Part model, mm, in its own coordinate system. A direction names the side the tool comes from. Round coordinates to 2 decimals unless told otherwise and drop trailing zeros. Write each loop counter-clockwise with the first axis right and the second up, starting at its lowest first coordinate (ties: lowest second). Pieces come first, ordered by that corner, then holes.
1) Saw through at D-D on y = -181. Write the cut outline in (x, z), and give its area (3 significant figures).
2) Which spindle directions (+Z, -Z, +X, -X, +Y, -Y) get a long thin tool onto all of the face, cutting with end or side? Do faces 4 (the flat face through (-100, -8.457, 10)), 5 (the flat face through (-102.851, 20.437, 9.86)), 6 (the flat face through (-12, -99, 20)). Say none if no direction does.
3) Drill centre lines: L1, parallel to Y at x = -142.5, z = 9; L2, parallel to X at y = -266, z = 16.5; L3, parallel to X at y = -232, z = 15.75. Where is each one in solid material? Low to high.
4) Saw through at C-C on x = -182.5. Write the cut outline in (y, z).
5) Saw through at B-B on y = -259. Write the cut outline in (x, z).
6) Flat gauge pins, fed straight in: pin 1 (1 mm diameter, centred on x = -67, z = 8, fed in from +Y); pin 2 (1 mm diameter, centred on y = -146, z = 13.5, fed in from +X); pin 3 (1 mm diameter, centred on y = -86.5, z = 14, fed in from +X); pin 4 (12 mm diameter, centred on x = -59.5, y = -207, fed in from +Z). Where does each tip first touch, or does it go through?
7) Pull direction X, two halves, no side cores. Call faces 1 (the flat face through (0, -36, 10)), 2 (the flat face through (8, 47.563, 10)), 3 (the flat face through (-8.927, -121.445, 9.86)): +X half, -X half, draft (parallel to the pull), parting line (faces both ways), or undercut.
8) Saw through at A-A on z = 16. Write the cut outline in (x, y).
```python
from build123d import *

# Parameters (mm, degrees)
BOSS_EXTRU_1_DEPTH = 20


with BuildPart() as part:
    # Esquisse1 → Boss.-Extru.1 (new body)
    with BuildSketch(Plane.XY):
        Polygon((-196.533735711, -8.457408384), (0, -8.457408384), (0, -64.477749577), (-85.505035831, -299.400904773), (-68.158030406, -299.400904773), (-23.296347582, -299.400904773), (58.442642683, -64.477749577), (15.742456943, 47.56293281), (0, 47.56293281), (-232.911164776, 20.29498163), (-207.234020919, 0), align=None)
        with BuildLine():
            ThreePointArc((-39.776845244, -207.826148347), (-17.410500422, -197.231497844), (-6.815849919, -219.597842666))
            Line((-6.815849919, -219.597842666), (-26.995897322, -276.102406082))
            ThreePointArc((-26.995897322, -276.102406082), (-49.362242144, -286.697056585), (-59.956892648, -264.330711763))
            Line((-59.956892648, -264.330711763), (-39.776845244, -207.826148347))
        make_face(mode=Mode.SUBTRACT)
        with BuildLine():
            ThreePointArc((1.304768326, -92.796753577), (23.671113149, -82.202103073), (34.265763652, -104.568447895))
            Line((34.265763652, -104.568447895), (14.085716249, -161.073011311))
            ThreePointArc((14.085716249, -161.073011311), (-8.280628573, -171.667661815), (-18.875279077, -149.301316992))
            Line((-18.875279077, -149.301316992), (1.304768326, -92.796753577))
        make_face(mode=Mode.SUBTRACT)
        Polygon((0, 30), (0, 0), (-190, 0), (-202.86096767, 11.137722401), align=None, mode=Mode.SUBTRACT)
    extrude(amount=BOSS_EXTRU_1_DEPTH)


solid = part.part
```
Completed:
1. outline: (-42.41, 0) - (17.9, 0) - (17.9, 20) - (-42.41, 20) - close
1. area: 1,210 mm2
2. face 4: +Z, -Z, -X
2. face 5: +Z, -Z
2. face 6: +Z, +X, -X, +Y, -Y
3. L1: y = -8.46 to 0, 16.75 to 30.88
3. L2: x = -73.35 to -60.46, -23.39 to -11.67
3. L3: x = -60.97 to -48.41, -11.25 to 0.16
4. outline: (-8.46, 0) - (0, 0) - (0, 20) - (-8.46, 20) - close; (13.03, 0) - (26.2, 0) - (26.2, 20) - (13.03, 20) - close
5. outline: (-70.8, 0) - (-58.05, 0) - (-58.05, 20) - (-70.8, 20) - close; (-20.89, 0) - (-9.24, 0) - (-9.24, 20) - (-20.89, 20) - close
6. pin 1: stops at y = 39.78
6. pin 2: stops at x = 30.25
6. pin 3: stops at x = 50.95
6. pin 4: passes through
7. face 1: -X half
7. face 2: draft
7. face 3: undercut
8. outline: (-232.91, 20.29) - (-196.53, -8.46) - (0, -8.46) - (0, -64.48) - (-85.51, -299.4) - (-23.3, -299.4) - (58.44, -64.48) - (15.74, 47.56) - (0, 47.56) - close; hole (-202.86, 11.14) - (-190, 0) - (0, 0) - (0, 30) - close; hole (-59.96, -264.33) arc R17.5 ccw to (-27, -276.1) - (-6.82, -219.6) arc R17.5 ccw to (-39.78, -207.83) - close; hole (-18.88, -149.3) arc R17.5 ccw to (14.09, -161.07) - (34.27, -104.57) arc R17.5 ccw to (1.3, -92.8) - close
